Part model, mm, in its own coordinate system. A direction names the side the tool comes from. Coordinates: 2 decimals unless noted, no trailing zeros. Write each loop counter-clockwise with the first axis right and the second up, starting at its lowest first coordinate (ties: lowest second). Pieces come first, ordered by that corner, then holes. Notation, with made-up numbers: (11, 82.25) -> (28, 82.25) arc R18 ccw to (28, 108.25) -> close; hole circle Ø11 at (71, 33.25). An arc over 180 degrees is marked (long way). Write item = value, one per line.
from build123d import *

# Parameters (mm, degrees)
BOSS_EXTRUDE1_DEPTH = 7.5
SKETCH2_R           = 1.75
BOSS_EXTRUDE2_DEPTH = 3
SKETCH3_W           = 5
SKETCH3_H           = 7.5
BOSS_EXTRUDE3_DEPTH = 3.5
CUT_EXTRUDE1_DEPTH  = 29.346075566
BOSS_EXTRUDE4_DEPTH = 3
RIB1_REACH          = 43.5
SKETCH7_WALL_W      = 89.242640688
SKETCH7_WALL_H      = 5.25255129
BOSS_EXTRUDE5_DEPTH = 2
CUT_EXTRUDE2_DEPTH  = 29.346075566


with BuildPart() as part:
    # Sketch1 → Boss-Extrude1 (new body)
    with BuildSketch(Plane.XY):
        with BuildLine():
            Line((-17.5, 0), (17.5, 0))
            Line((17.5, 0), (17.5, 17.5))
            Line((17.5, 17.5), (12.5, 17.5))
            ThreePointArc((12.5, 17.5), (0, 5), (-12.5, 17.5))
            Line((-12.5, 17.5), (-17.5, 17.5))
            Line((-17.5, 17.5), (-17.5, 0))
        make_face()
    extrude(amount=BOSS_EXTRUDE1_DEPTH)

    # Sketch2 → Boss-Extrude2 (add)
    # profile 1 of 2: a face of its own
    with BuildSketch(Plane(origin=(0, 0, 0), x_dir=(-1, 0, 0), z_dir=(0, 0, -1))):
        with BuildLine():
            Line((-8.5, 14), (-14, 14))
            ThreePointArc((-14, 14), (-17.5, 17.5), (-14, 21))
            Line((-14, 21), (-8.5, 21))
            ThreePointArc((-8.5, 21), (-5, 17.5), (-8.5, 14))
        make_face()
        with Locations((-8.5, 17.5)):
            Circle(SKETCH2_R, mode=Mode.SUBTRACT)
    # profile 2 of 2: a face of its own
    with BuildSketch(Plane(origin=(0, 0, 0), x_dir=(-1, 0, 0), z_dir=(0, 0, -1))):
        with BuildLine():
            Line((8.5, 14), (14, 14))
            ThreePointArc((14, 14), (17.5, 17.5), (14, 21))
            Line((14, 21), (8.5, 21))
            ThreePointArc((8.5, 21), (5, 17.5), (8.5, 14))
        make_face()
        with Locations(Location((8.5, 17.5, 0), (0, 0, 180))):
            Circle(SKETCH2_R, mode=Mode.SUBTRACT)
    extrude(amount=BOSS_EXTRUDE2_DEPTH)

    # Sketch3 → Boss-Extrude3 (add)
    with BuildSketch(Plane(origin=(0, 17.5, 0), x_dir=(1, 0, 0), z_dir=(0, 1, 0))):
        with Locations((15, -3.75)):
            Rectangle(SKETCH3_W, SKETCH3_H)
        with Locations((-15, -3.75)):
            Rectangle(SKETCH3_W, SKETCH3_H)
    extrude(amount=BOSS_EXTRUDE3_DEPTH)

    # Sketch4 → Cut-Extrude1 (cut, through all)
    with BuildSketch(Plane(origin=(0, 0, 0), x_dir=(-1, 0, 0), z_dir=(0, 0, -1))):
        with BuildLine():
            Line((17.5, 21), (17.5, 17.5))
            ThreePointArc((17.5, 17.5), (16.474873734, 19.974873734), (14, 21))
            Line((14, 21), (17.5, 21))
        make_face()
    cut_extrude1 = extrude(amount=-CUT_EXTRUDE1_DEPTH, mode=Mode.SUBTRACT)

    # Sketch5 → Boss-Extrude4 (add)
    with BuildSketch(Plane(origin=(0, 0, 0), x_dir=(-1, 0, 0), z_dir=(0, 0, -1))):
        with BuildLine():
            Line((14, 14), (17.5, 14))
            Line((17.5, 14), (17.5, 17.5))
            ThreePointArc((17.5, 17.5), (16.474873734, 15.025126266), (14, 14))
        make_face()
    boss_extrude4 = extrude(amount=BOSS_EXTRUDE4_DEPTH)

    # Mirror1: Cut-Extrude1, Boss-Extrude4 across plane
    add(cut_extrude1.mirror(Plane(origin=(0, 0, 0), x_dir=(0, 0, 1), z_dir=(1, 0, 0))), mode=Mode.SUBTRACT)
    add(boss_extrude4.mirror(Plane(origin=(0, 0, 0), x_dir=(0, 0, 1), z_dir=(1, 0, 0))))

    # Sketch7 wall → Rib1 (add, up to next)
    with BuildSketch(Plane(origin=(17.5, 12.5, -1.5), x_dir=(0, -0.707106781187, 0.707106781187), z_dir=(0, -0.707106781187, -0.707106781187)), mode=Mode.PRIVATE) as rib1_sk1:
        with Locations((0, 2.626275645)):
            Rectangle(SKETCH7_WALL_W, SKETCH7_WALL_H)
    rib1_tool1 = extrude(rib1_sk1.sketch, amount=-RIB1_REACH, mode=Mode.PRIVATE) - part.part
    rib1 = rib1_tool1.solids().sort_by_distance((17.5, 12.5, -1.5))[0]
    add(rib1)

    # Mirror2: Rib1 across plane
    add(rib1.mirror(Plane(origin=(0, 0, 0), x_dir=(0, 0, 1), z_dir=(1, 0, 0))))

    # Sketch8 → Boss-Extrude5 (add)
    with BuildSketch(Plane(origin=(-12.24744871, 0, 0), x_dir=(0, 0, -1), z_dir=(1, 0, 0))):
        Polygon((3, 14), (0, 11), (0, 14), align=None)
    boss_extrude5 = extrude(amount=BOSS_EXTRUDE5_DEPTH)

    # Sketch9 → Cut-Extrude2 (cut, through all)
    with BuildSketch(Plane.XY):
        with BuildLine():
            Line((-10.24744871, 14), (-12, 14))
            ThreePointArc((-12, 14), (-11.437327901, 12.456436727), (-10.677078252, 11))
            Line((-10.677078252, 11), (-10.24744871, 11))
            Line((-10.24744871, 11), (-10.24744871, 14))
        make_face()
    cut_extrude2 = extrude(amount=-CUT_EXTRUDE2_DEPTH, mode=Mode.SUBTRACT)

    # Mirror3: Boss-Extrude5, Cut-Extrude2 across plane
    add(boss_extrude5.mirror(Plane(origin=(0, 0, 0), x_dir=(0, 0, 1), z_dir=(1, 0, 0))))
    add(cut_extrude2.mirror(Plane(origin=(0, 0, 0), x_dir=(0, 0, 1), z_dir=(1, 0, 0))), mode=Mode.SUBTRACT)


solid = part.part
Q1. Saw through at B-B on x = 9. Give the cut face in (y, z).
Model answer:
outline = (0, 0) -> (8.83, 0) -> (8.83, 7.5) -> (0, 7.5) -> close; (14, -3) -> (15.82, -3) -> (15.82, 0) -> (14, 0) -> close; (19.18, -3) -> (21, -3) -> (21, 0) -> (19.18, 0) -> close
Q2. Pin check, flat tips, straight feed: pin 1 (1 mm diameter, centred on y = 19, z = 2, fed in from +X); pin 2 (5.5 mm diameter, centred on x = -8.5, y = 17.5, fed in from +Z); pin 3 (1 mm diameter, centred on x = 7, z = -1.5, fed in from +Y). Stop position of each tip, or through.
Model answer:
pin_1 = 17.35
pin_2 = 0
pin_3 = 20.85
Q3. Saw through at D-D on y = 4. Give the cut face in (x, z), and give its area (4 significant figures).
Model answer:
outline = (-17.5, 0) -> (17.5, 0) -> (17.5, 7.5) -> (-17.5, 7.5) -> close
area = 262.5 mm²
Q4. Mould opens along X. For faces 6 (the face through (11.8, 21, -0.2)), 7 (the face through (17.5, 10, 3)), 8 (the face through (-10, 14, -1)) say: released by +X, released by -X, zero draft, split by the parting line, or undercut.
Model answer:
face_6 = zero draft
face_7 = released by +X
face_8 = undercut
Q5. Saw through at C-C on z = 2.25. Give the cut face in (x, y), and give its area (3 significant figures).
Model answer:
outline = (-17.5, 0) -> (17.5, 0) -> (17.5, 17.5) arc R3.5 ccw to (14, 21) -> (12.5, 21) -> (12.5, 17.5) arc R12.5 cw to (-12.5, 17.5) -> (-12.5, 21) -> (-14, 21) arc R3.5 ccw to (-17.5, 17.5) -> close
area = 397 mm²
Q6. Saw through at A-A on y = 7.5. Give the cut face in (x, z).
Model answer:
outline = (-17.5, 0) -> (-7.5, 0) -> (-7.5, 7.5) -> (-17.5, 7.5) -> close; (7.5, 0) -> (17.5, 0) -> (17.5, 7.5) -> (7.5, 7.5) -> close
Q7. Probe line 1 (Y direction, x = 8.5, z = -1.6); line 2 (Z direction, x = -9, y = 14.75); line 3 (X direction, y = 18.5, z = -1). List the from-to ranges inside material, lowest first. Write a range as from..to.
Model answer:
line_1 = 14..15.75, 19.25..21
line_2 = -3..0
line_3 = -17.35..-9.94, -7.06..-5.15, 5.15..7.06, 9.94..17.35
Q8. Which spindle directions (+Z, -Z, +X, -X, +Y, -Y) get a long thin tool onto all of the face, cutting with end or side? Do faces 1 (the face through (12.5, 19, 4)), 2 (the face through (0, 4, 0)), 3 (the face through (11, 18, -3)), 4 (the face through (-5, 17.6, -1.5)), 5 (the face through (0, 0, 4)). Say none if no direction does.
Model answer:
face_1 = +Z, +Y
face_2 = -Z, +X, -X, -Y
face_3 = -Z, +X, -X, +Y, -Y
face_4 = +Z, -Z
face_5 = +Z, -Z, +X, -X, -Y
